Build history of the part. All positions in model axes, mm. Face numbers are marked on the shaded views. A direction names the side the tool comes from. Coordinates: 2 decimals unless noted, no trailing zeros. Write each loop counter-clockwise with the first axis right and the second up, starting at its lowest first coordinate (ties: lowest second). Pieces come first, ordered by that corner, then holes.
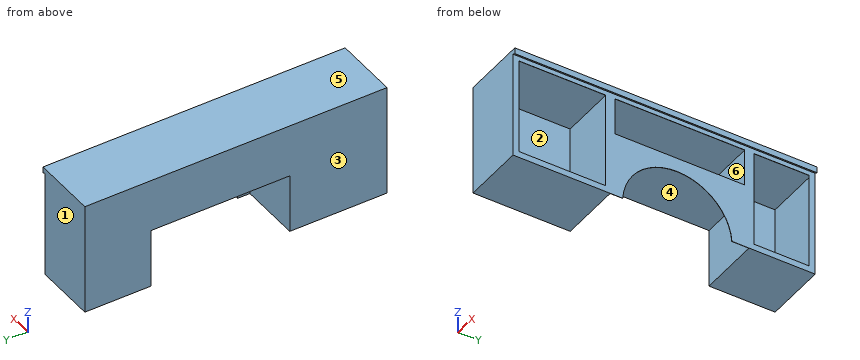
from build123d import *

# Parameters (mm, degrees)
F0_W      = 508
F0_H      = 914.4
F1_DEPTH  = 2470.15
F2_W      = 704.85
F2_H      = 787.4
F2_W_2    = 1060.45
F2_H_2    = 304.8
F2_W_3    = 450.85
F3_DEPTH  = 505.8918
F4_W      = 503.7836
F4_H      = 704.85
F5_DEPTH  = 48.6918
F6_W      = 503.7836
F6_H      = 704.85
F7_DEPTH  = 48.6918
F8_W      = 503.7836
F8_H      = 884.7836
F9_DEPTH  = 48.6918
F10_W     = 503.7836
F10_H     = 884.7836
F11_DEPTH = 37.0459
F12_W     = 503.7836
F12_H     = 1060.45
F13_DEPTH = 48.6918
F14_W     = 503.7836
F14_H     = 1060.45
F15_DEPTH = 48.6918
F16_W     = 503.7836
F16_H     = 402.1836
F17_DEPTH = 37.0459
F18_W     = 503.7836
F18_H     = 402.1836
F19_DEPTH = 37.0459
F20_W     = 503.7836
F20_H     = 450.85
F21_DEPTH = 48.6918
F22_W     = 503.7836
F22_H     = 450.85
F23_DEPTH = 48.6918
F24_W     = 503.7836
F24_H     = 884.7836
F25_DEPTH = 37.0459
F26_W     = 503.7836
F26_H     = 884.7836
F27_DEPTH = 48.6918
F28_W     = 505.8918
F28_H     = 1134.5418
F29_DEPTH = 482.6
F31_DEPTH = 508.001
F33_DEPTH = 2470.15
F34_R     = 0.508


with BuildPart() as f1:
    # F0 (on Front) → F1 (new body)
    with BuildSketch(Plane.XZ):
        Rectangle(F0_W, F0_H)
    extrude(amount=-F1_DEPTH)

    # F2 (on face) → F3 (cut)
    with BuildSketch(Plane.YZ.offset(254)):
        with Locations((403.225, -12.7)):
            Rectangle(F2_W, F2_H)
        with Locations((1362.075, 228.6)):
            Rectangle(F2_W_2, F2_H_2)
        with Locations((2193.925, -12.7)):
            Rectangle(F2_W_3, F2_H)
    extrude(amount=-F3_DEPTH, mode=Mode.SUBTRACT)

    # F4 (on face) → F5 (cut)
    with BuildSketch(Plane.XY.offset(-406.4)):
        with Locations((0, 403.225)):
            Rectangle(F4_W, F4_H)
    extrude(amount=-F5_DEPTH, mode=Mode.SUBTRACT)

    # F6 (on face) → F7 (cut)
    with BuildSketch(Plane(origin=(0, 0, 381), x_dir=(1, 0, 0), z_dir=(0, 0, -1))):
        with Locations((0, -403.225)):
            Rectangle(F6_W, F6_H)
    extrude(amount=-F7_DEPTH, mode=Mode.SUBTRACT)

    # F8 (on face) → F9 (cut)
    with BuildSketch(Plane(origin=(0, 50.8, 0), x_dir=(-1, 0, 0), z_dir=(0, 1, 0))):
        with Locations((0, -12.7)):
            Rectangle(F8_W, F8_H)
    extrude(amount=-F9_DEPTH, mode=Mode.SUBTRACT)

    # F10 (on face) → F11 (cut)
    with BuildSketch(Plane.XZ.offset(-755.65)):
        with Locations((0, -12.7)):
            Rectangle(F10_W, F10_H)
    extrude(amount=-F11_DEPTH, mode=Mode.SUBTRACT)

    # F12 (on face) → F13 (cut)
    with BuildSketch(Plane.XY.offset(76.2)):
        with Locations((0, 1362.075)):
            Rectangle(F12_W, F12_H)
    extrude(amount=-F13_DEPTH, mode=Mode.SUBTRACT)

    # F14 (on face) → F15 (cut)
    with BuildSketch(Plane(origin=(0, 0, 381), x_dir=(1, 0, 0), z_dir=(0, 0, -1))):
        with Locations((0, -1362.075)):
            Rectangle(F14_W, F14_H)
    extrude(amount=-F15_DEPTH, mode=Mode.SUBTRACT)

    # F16 (on face) → F17 (cut)
    with BuildSketch(Plane(origin=(0, 831.85, 0), x_dir=(-1, 0, 0), z_dir=(0, 1, 0))):
        with Locations((0, 228.6)):
            Rectangle(F16_W, F16_H)
    extrude(amount=-F17_DEPTH, mode=Mode.SUBTRACT)

    # F18 (on face) → F19 (cut)
    with BuildSketch(Plane.XZ.offset(-1892.3)):
        with Locations((0, 228.6)):
            Rectangle(F18_W, F18_H)
    extrude(amount=-F19_DEPTH, mode=Mode.SUBTRACT)

    # F20 (on face) → F21 (cut)
    with BuildSketch(Plane.XY.offset(-406.4)):
        with Locations((0, 2193.925)):
            Rectangle(F20_W, F20_H)
    extrude(amount=-F21_DEPTH, mode=Mode.SUBTRACT)

    # F22 (on face) → F23 (cut)
    with BuildSketch(Plane(origin=(0, 0, 381), x_dir=(1, 0, 0), z_dir=(0, 0, -1))):
        with Locations((0, -2193.925)):
            Rectangle(F22_W, F22_H)
    extrude(amount=-F23_DEPTH, mode=Mode.SUBTRACT)

    # F24 (on face) → F25 (cut)
    with BuildSketch(Plane(origin=(0, 1968.5, 0), x_dir=(-1, 0, 0), z_dir=(0, 1, 0))):
        with Locations((0, -12.7)):
            Rectangle(F24_W, F24_H)
    extrude(amount=-F25_DEPTH, mode=Mode.SUBTRACT)

    # F26 (on face) → F27 (cut)
    with BuildSketch(Plane.XZ.offset(-2419.35)):
        with Locations((0, -12.7)):
            Rectangle(F26_W, F26_H)
    extrude(amount=-F27_DEPTH, mode=Mode.SUBTRACT)

    # F28 (on face) → F29 (cut)
    with BuildSketch(Plane(origin=(0, 0, -457.2), x_dir=(1, 0, 0), z_dir=(0, 0, -1))):
        with Locations((-1.0541, -1362.075)):
            Rectangle(F28_W, F28_H)
    extrude(amount=-F29_DEPTH, mode=Mode.SUBTRACT)

    # F30 (on face) → F31 (cut, through all)
    with BuildSketch(Plane.YZ.offset(254)):
        with BuildLine():
            Line((896.4041, -457.2), (1789.6459, -457.2))
            ThreePointArc((1789.6459, -457.2), (1343.025, -38.1), (896.4041, -457.2))
        make_face()
    extrude(amount=-F31_DEPTH, mode=Mode.SUBTRACT)

    # F32 (on face) → F33 (join, through all)
    with BuildSketch(Plane.XZ):
        Polygon((277.0862247403, 459.3082), (-254, 459.3082), (-254, 457.2), (254, 457.2), (254, 419.1), (277.0862247403, 408.5082), align=None)
    extrude(amount=-F33_DEPTH)

    # F34
    f34_edges = [f1.edges().sort_by_distance(p)[0] for p in [
        (277.086225, 1235.075, 408.5082),
    ]]
    fillet(f34_edges, radius=F34_R)


solid = f1.part
(1) Flat gauge pins, fed straight in: P1, Ø4, axis at x = 32.5, y = 1639, coming from the -Z side; P2, Ø1.5, axis at y = 1765, z = 283.5, coming from the +X side. Where does each tip first touch, or does it go through?
(2) 3-axis set-ups, long thin cutter, end or side, ignore diameter. For the marked faces 4, 5 and 6: which of +Z, -Z, +X, -X, +Y, -Y reach the whole face in a straight line?
(3) Slice it at B-B, the plane x = -35.5. List the corners of the cut face in (y, z).
(4) Slice it at D-D, the plane z = -348. List the corners of the cut face in (x, y).
(5) Probe L1, parallel to Y at x = -119, z = 97; L2, parallel to Y at x = 253, z = 9; L3, parallel to Z at x = 76.5, y = 1581. List the from-to ranges inside material, lowest first.
(6) Slice it at C-C, the plane y = 1831.5. List the corners of the cut face in (x, z), and give its area (3 significant figures).
(7) Two-plate mould, pull along Y, no slides. Class the marked faces 1, 2 and 3: pulls with the +Y half, pulls with the -Y half, needs draft (parallel to the pull), parting line crosses it, or undercut.
(8) Slice it at A-A, the plane z = 198.5. List the corners of the cut face in (x, y).
Results:
1. P1: stops at z = 25.4
1. P2: stops at x = -251.89
2. face 4: -Z, -X
2. face 5: +Z, +X, -X, +Y, -Y
2. face 6: none
3. outline: (0, -457.2) - (794.8, -457.2) - (794.8, 25.4) - (1929.35, 25.4) - (1929.35, -457.2) - (2470.15, -457.2) - (2470.15, 459.31) - (0, 459.31) - close; hole (2.11, -455.09) - (792.7, -455.09) - (792.7, 429.69) - (2.11, 429.69) - close; hole (794.8, 27.51) - (1929.35, 27.51) - (1929.35, 429.69) - (794.8, 429.69) - close; hole (1931.45, -455.09) - (2468.04, -455.09) - (2468.04, 429.69) - (1931.45, 429.69) - close
4. outline: (-254, 0) - (254, 0) - (254, 50.8) - (251.89, 50.8) - (251.89, 2.11) - (-251.89, 2.11) - (-251.89, 792.7) - (251.89, 792.7) - (251.89, 755.65) - (254, 755.65) - (254, 917.19) - (251.89, 917.19) - (251.89, 794.8) - (-254, 794.8) - close; (-254, 1929.35) - (251.89, 1929.35) - (251.89, 1768.86) - (254, 1768.86) - (254, 1968.5) - (251.89, 1968.5) - (251.89, 1931.45) - (-251.89, 1931.45) - (-251.89, 2468.04) - (251.89, 2468.04) - (251.89, 2419.35) - (254, 2419.35) - (254, 2470.15) - (-254, 2470.15) - close
5. L1: y = 0 to 2.11, 792.7 to 794.8, 1929.35 to 1931.45, 2468.04 to 2470.15
5. L2: y = 0 to 50.8, 755.65 to 1968.5, 2419.35 to 2470.15
5. L3: z = 25.4 to 27.51, 429.69 to 459.31
6. outline: (-254, 25.4) - (251.89, 25.4) - (251.89, -457.2) - (254, -457.2) - (254, 76.2) - (251.89, 76.2) - (251.89, 27.51) - (-251.89, 27.51) - (-251.89, 429.69) - (251.89, 429.69) - (251.89, 381) - (254, 381) - (254, 419.1) - (276.37, 408.84) arc R0.51 ccw to (277.09, 409.3) - (277.09, 459.31) - (-254, 459.31) - close
6. area: 19,200 mm2
7. face 1: pulls with the +Y half
7. face 2: undercut
7. face 3: needs draft
8. outline: (-254, 0) - (254, 0) - (254, 50.8) - (251.89, 50.8) - (251.89, 2.11) - (-251.89, 2.11) - (-251.89, 792.7) - (251.89, 792.7) - (251.89, 755.65) - (254, 755.65) - (254, 831.85) - (251.89, 831.85) - (251.89, 794.8) - (-251.89, 794.8) - (-251.89, 1929.35) - (251.89, 1929.35) - (251.89, 1892.3) - (254, 1892.3) - (254, 1968.5) - (251.89, 1968.5) - (251.89, 1931.45) - (-251.89, 1931.45) - (-251.89, 2468.04) - (251.89, 2468.04) - (251.89, 2419.35) - (254, 2419.35) - (254, 2470.15) - (-254, 2470.15) - close
